from build123d import *

# Parameters (mm, degrees)
BOSS_EXTRUDE1_DEPTH = 3
SKETCH3_W           = 25
SKETCH3_H           = 7
BOSS_EXTRUDE2_DEPTH = 4
SKETCH2_R           = 1.592288308
CUT_EXTRUDE1_DEPTH  = 10
FILLET1_R           = 3


with BuildPart() as part:
    # Sketch1 → Boss-Extrude1 (new body)
    with BuildSketch(Plane.XY):
        Polygon((-12.549665985, 17.237823834), (-5.049665985, 17.237823834), (-5.049665985, 24.237823834), (-30.049665985, 24.237823834), (-30.049665985, 17.237823834), (-22.549665985, 17.237823834), (-22.549665985, -28.68448974), (-12.549665985, -28.68448974), align=None)
        with BuildLine():
            Line((-19.349665985, -23.68448974), (-19.349665985, -6.438362401))
            ThreePointArc((-19.349665985, -6.438362401), (-17.549665985, -4.638362401), (-15.749665985, -6.438362401))
            Line((-15.749665985, -6.438362401), (-15.749665985, -23.68448974))
            ThreePointArc((-15.749665985, -23.68448974), (-17.549665985, -25.48448974), (-19.349665985, -23.68448974))
        make_face(mode=Mode.SUBTRACT)
    extrude(amount=BOSS_EXTRUDE1_DEPTH)

    # Sketch3 → Boss-Extrude2 (add)
    with BuildSketch(Plane.XY.offset(3)):
        with Locations((-17.549665985, 20.737823834)):
            Rectangle(SKETCH3_W, SKETCH3_H)
    extrude(amount=BOSS_EXTRUDE2_DEPTH)

    # Sketch2 → Cut-Extrude1 (cut)
    with BuildSketch(Plane.XY):
        with Locations((-25.049665985, 20.737823834)):
            Circle(SKETCH2_R)
        with Locations((-10.049665985, 20.737823834)):
            Circle(SKETCH2_R)
    extrude(amount=CUT_EXTRUDE1_DEPTH, mode=Mode.SUBTRACT)

    # Fillet1
    fillet1_edges = [part.edges().sort_by_distance(p)[0] for p in [
        (-5.049665985, 17.237823834, 3.5),
        (-12.549665985, 17.237823834, 1.5),
        (-12.549665985, -28.68448974, 1.5),
        (-22.549665985, -28.68448974, 1.5),
        (-22.549665985, 17.237823834, 1.5),
        (-30.049665985, 17.237823834, 3.5),
        (-30.049665985, 24.237823834, 3.5),
        (-5.049665985, 24.237823834, 3.5),
        (-17.549665985, 17.237823834, 3),
    ]]
    fillet(fillet1_edges, radius=FILLET1_R)


solid = part.part
Check sheet for the modelled part. Datum: model origin and axes. Units: mm. A direction names the side the tool comes from. Round coordinates to 2 decimals unless told otherwise and drop trailing zeros. Order: outer loops, then holes, each group sorted by start corner. A loop starts at its lowest first (then second) coordinate and runs counter-clockwise, first axis right, second up.
(1) Cross-section at A-A, the plane y = -8. Enter the section's corners in (x, z), and give its area (3 significant figures).
(2) Draft check along Y on faces 1 (the cylindrical face through (-9.19, 22.08, 3.45)), 2 (the flat face through (-20, -7, 3)), 3 (the cylindrical face through (-21.648, -27.829, 1.521)). Enter one of: pulls with the +Y half, pulls with the -Y half, needs draft (parallel to the pull), parting line crosses it, or undercut.
(3) Cross-section at D-D, the plane z = 5.5. Enter the section's corners in (x, y), and give its area (3 significant figures).
(4) Cross-section at B-B, the plane x = -10.5. Enter the section's corners in (y, z), and give its area (3 significant figures).
(5) Go/stop test with flat-tipped pins: P1, Ø8, axis at x = -17, y = -18, coming from the +Z side; P2, Ø3.5, axis at y = -13.5, z = 1.5, coming from the -X side; P3, Ø0.9, axis at y = -13, z = 1, coming from the +X side. Record where each tip stops, or that it passes through.
(6) Cross-section at C-C, the plane z = 1. Enter the section's corners in (x, y), and give its area (3 significant figures).
(7) Scan lines: probe 1 along X at (y, z) = (-16, 0.75); probe 2 along X at (y, z) = (20, 2.5); probe 3 along X at (y, z) = (11, 2.75). Record each from-to range of solid material in increasing order.
(8) Access from +Z, -Z, +X, -X, +Y, -Y to the whole of each face (thin tool, end or side, straight path). Record for faces 4 (the cylindrical face through (-17.59, -4.64, 1.48)), 5 (the flat face through (-17.6, 17.238, 6.3)), 6 (the flat face through (-18, 21, 7)), 7 (the flat face through (-18, -28.684, 1)), 8 (the flat face through (-22.55, -5, 1)).
Check sheet entries:
1. outline: (-22.55, 0) - (-19.35, 0) - (-19.35, 3) - (-22.55, 3) - close; (-15.75, 0) - (-12.55, 0) - (-12.55, 3) - (-15.75, 3) - close
1. area: 19.2 mm2
2. face 1: undercut
2. face 2: needs draft
2. face 3: pulls with the -Y half
3. outline: (-30.05, 20.24) arc R3 ccw to (-27.05, 17.24) - (-25.55, 17.24) arc R3 cw to (-25.05, 17.2) - (-10.05, 17.2) arc R3 cw to (-9.55, 17.24) - (-8.05, 17.24) arc R3 ccw to (-5.05, 20.24) - (-5.05, 21.24) arc R3 ccw to (-8.05, 24.24) - (-27.05, 24.24) arc R3 ccw to (-30.05, 21.24) - close; hole circle Ø3.18 at (-25.05, 20.74); hole circle Ø3.18 at (-10.05, 20.74)
3. area: 152 mm2
4. outline: (17.08, 0) - (19.21, 0) - (19.21, 7) - (17.24, 7) - (17.24, 6) arc R3 cw to (17.08, 5.05) - close; (22.27, 0) - (24.24, 0) - (24.24, 7) - (22.27, 7) - close
4. area: 28.4 mm2
5. P1: stops at z = 3
5. P2: stops at x = -22.55
5. P3: stops at x = -12.55
6. outline: (-30.05, 20.24) arc R3 ccw to (-27.05, 17.24) - (-25.55, 17.24) arc R3 cw to (-22.55, 14.24) - (-22.55, -25.68) arc R3 ccw to (-19.55, -28.68) - (-15.55, -28.68) arc R3 ccw to (-12.55, -25.68) - (-12.55, 14.24) arc R3 cw to (-9.55, 17.24) - (-8.05, 17.24) arc R3 ccw to (-5.05, 20.24) - (-5.05, 21.24) arc R3 ccw to (-8.05, 24.24) - (-27.05, 24.24) arc R3 ccw to (-30.05, 21.24) - close; hole circle Ø3.18 at (-25.05, 20.74); hole (-19.35, -23.68) arc R1.8 ccw to (-15.75, -23.68) - (-15.75, -6.44) arc R1.8 ccw to (-19.35, -6.44) - close; hole circle Ø3.18 at (-10.05, 20.74)
6. area: 538 mm2
7. probe 1: x = -22.55 to -19.35, -15.75 to -12.55
7. probe 2: x = -30.04 to -26.46, -23.64 to -11.46, -8.64 to -5.06
7. probe 3: x = -22.55 to -12.55
8. face 4: +Z, -Z
8. face 5: +Z, -Y
8. face 6: +Z, +X, -X, +Y, -Y
8. face 7: +Z, -Z, +X, -X, -Y
8. face 8: +Z, -Z, -X, -Y
